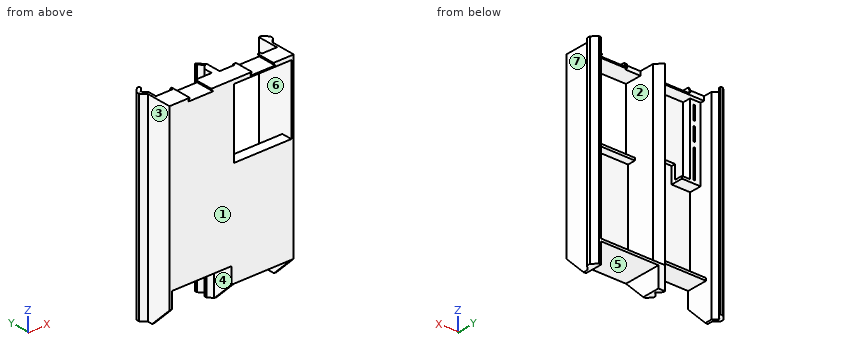
```python
from build123d import *

# Parameters (mm, degrees)
EXTRUDE_1_DEPTH       = 200
SKETCH_2_W            = 148
SKETCH_2_H            = 194
CUT_EXTRUDE_1_DEPTH   = 44
SKETCH_3_W            = 8
SKETCH_3_H            = 194
EXTRUDE_1_2_DEPTH     = 44
CUT_EXTRUDE_2_DEPTH   = 222.580685079
CUT_EXTRUDE_3_DEPTH   = 219.876677606
MOVE_FACE_1_BY        = 2
MOVE_FACE_1_2_BY      = 2
CUT_EXTRUDE_4_DEPTH   = 222.580685079
CUT_EXTRUDE_5_DEPTH   = 16.171573
MOVE_FACE_2_BY        = 45
MOVE_START            = -217
MOVE_FACE_4_DEPTH     = 20
SKETCH_10_W           = 71
SKETCH_10_H           = 47
CUT_EXTRUDE_6_DEPTH   = 25
SKETCH_11_W           = 69
SKETCH_11_H           = 26
CUT_EXTRUDE_7_DEPTH   = 45
CUT_EXTRUDE_8_DEPTH   = 45
CHAMFER_1_SIZE        = 25
CUT_EXTRUDE_9_REACH   = 264.393
SKETCH_13_W           = 71
SKETCH_13_H           = 85
SKETCH_14_W           = 71
SKETCH_14_H           = 3
EXTRUDE_2_DEPTH       = 10
CUT_EXTRUDE_10_DEPTH  = 16.171572875
SKETCH_16_W           = 18.7
SKETCH_16_H           = 5
CUT_EXTRUDE_11_DEPTH  = 4.2
SKETCH_17_W           = 69
SKETCH_17_H           = 90
EXTRUDE_3_DEPTH       = 15
SKETCH_18_W           = 56
SKETCH_18_H           = 87
CUT_EXTRUDE_12_DEPTH  = 10
CUT_EXTRUDE_13_REACH  = 262.298
SKETCH_19_W           = 36
SKETCH_19_H           = 34
SKETCH_21_W           = 2
SKETCH_21_H           = 17
SKETCH_21_H_2         = 35
CUT_EXTRUDE_1_2_DEPTH = 7
MOVE_FACE_5_BY        = 3


# Read off the part's stored shape, not the designer's step: 移动面4
with BuildPart() as part:
    # 草图1 → Extrude 1 (new body)
    with BuildSketch(Plane.XY):
        Polygon((77, 0), (-77, 0), (-77, 31), (-83, 37), (-83, 41), (-77, 47), (77, 47), (83, 41), (83, 37), (77, 31), align=None)
    extrude(amount=-EXTRUDE_1_DEPTH)

    # 草图2 → Cut-Extrude 1 (cut)
    with BuildSketch(Plane(origin=(0, 47, 0), x_dir=(1, 0, 0), z_dir=(0, 1, 0))):
        with Locations((0, 100)):
            Rectangle(SKETCH_2_W, SKETCH_2_H)
    extrude(amount=-CUT_EXTRUDE_1_DEPTH, mode=Mode.SUBTRACT)

    # 草图3 → Extrude 1 2 (add)
    with BuildSketch(Plane(origin=(0, 3, 0), x_dir=(1, 0, 0), z_dir=(0, 1, 0))):
        with Locations((-1, 100)):
            Rectangle(SKETCH_3_W, SKETCH_3_H)
    extrude(amount=EXTRUDE_1_2_DEPTH)

    # 草图6 → 切除-拉伸2 (cut, through all)
    with BuildSketch(Plane.XY):
        Polygon((-74, 47), (-74, 44.343145751), (-79, 39.343145751), (-79, 38.656854249), (-74, 33.656854249), (-74, 26), (-5, 26), (-5, 33.656854249), (0, 38.656854249), (0, 39.343145751), (-5, 44.343145751), (-5, 47), align=None)
    extrude(amount=-CUT_EXTRUDE_2_DEPTH, mode=Mode.SUBTRACT)

    # 草图7 → 切除-拉伸3 (cut, through all)
    with BuildSketch(Plane.XY.offset(-197)):
        Polygon((-4.828427125, 47), (3, 39.171572875), (74, 39.171572875), (74, 47), (3, 47), align=None)
    extrude(amount=CUT_EXTRUDE_3_DEPTH, mode=Mode.SUBTRACT)

    # Move Face 1: a face moved outward by 2.0
    extrude(part.faces().sort_by_distance((-39.5, 14.5, -3))[0], amount=MOVE_FACE_1_BY, dir=(0, 0, -1))

    # Move Face 1 2: a face moved outward by 2.0
    extrude(part.faces().sort_by_distance((38.5, 21.085786438, -3))[0], amount=MOVE_FACE_1_2_BY, dir=(0, 0, -1))

    # 草图8 → 切除-拉伸4 (cut, through all)
    with BuildSketch(Plane.XZ):
        Polygon((-51.883419246, 0), (-53.904145188, -3.5), (-23.095854812, -3.5), (-25.116580754, 0), align=None)
        Polygon((25.116580754, 0), (51.883419246, 0), (53.904145188, -3.5), (23.095854812, -3.5), align=None)
    extrude(amount=-CUT_EXTRUDE_4_DEPTH, mode=Mode.SUBTRACT)

    # 草图9 → 切除-拉伸5 (cut)
    with BuildSketch(Plane(origin=(0, 39.171572875, 0), x_dir=(1, 0, 0), z_dir=(0, 1, 0))):
        Polygon((26.616580754, 0), (24.595854812, 3.5), (55.404145188, 3.5), (53.383419246, 0), (74, 0), (74, 5), (3, 5), (3, 0), align=None)
        Polygon((-55.404145188, 3.5), (-24.595854812, 3.5), (-26.616580754, 0), (-5, 0), (-5, 5), (-74, 5), (-74, 0), (-53.383419246, 0), align=None)
    extrude(amount=-CUT_EXTRUDE_5_DEPTH, mode=Mode.SUBTRACT)

    # Move Face 2: a face moved outward by 45.0
    extrude(part.faces().sort_by_distance((10.164079255, 20.448401084, -200))[0], amount=MOVE_FACE_2_BY, dir=(0, 0, -1))

    # Move Face 4 outline → Move Face 4 (cut)
    with BuildSketch(Plane.XY.offset(MOVE_START)):
        Polygon((74, 3), (74, 47), (-4.828427125, 47), (3, 39.171572875), (3, 3), align=None)
    extrude(amount=MOVE_FACE_4_DEPTH, mode=Mode.SUBTRACT)

    # 草图10 → 切除-拉伸6 (cut)
    with BuildSketch(Plane(origin=(0, 0, -245), x_dir=(-1, 0, 0), z_dir=(0, 0, -1))):
        with Locations((-38.5, 23.5)):
            Rectangle(SKETCH_10_W, SKETCH_10_H)
    extrude(amount=-CUT_EXTRUDE_6_DEPTH, mode=Mode.SUBTRACT)

    # 草图11 → 切除-拉伸7 (cut)
    with BuildSketch(Plane(origin=(0, 0, -245), x_dir=(-1, 0, 0), z_dir=(0, 0, -1))):
        with Locations((39.5, 13)):
            Rectangle(SKETCH_11_W, SKETCH_11_H)
    extrude(amount=-CUT_EXTRUDE_7_DEPTH, mode=Mode.SUBTRACT)

    # 草图12 → 切除-拉伸8 (cut)
    with BuildSketch(Plane(origin=(0, 0, -245), x_dir=(-1, 0, 0), z_dir=(0, 0, -1))):
        Polygon((5, 0), (0, 0), (0, 25.656854249), (5, 30.656854249), align=None)
    extrude(amount=-CUT_EXTRUDE_8_DEPTH, mode=Mode.SUBTRACT)

    # 倒角1
    chamfer_1_edges = [part.edges().sort_by_distance(p)[0] for p in [
        (-75.5, 0, -245),
        (1.5, 0, -245),
        (75.5, 0, -245),
    ]]
    chamfer(chamfer_1_edges, length=CHAMFER_1_SIZE)

    # 草图13 → 切除-拉伸9 (cut, up to next)
    with BuildSketch(Plane(origin=(0, 3, 0), x_dir=(1, 0, 0), z_dir=(0, 1, 0)), mode=Mode.PRIVATE) as cut_extrude_9_sk1:
        with Locations((38.5, 47.5)):
            Rectangle(SKETCH_13_W, SKETCH_13_H)
    cut_extrude_9_tool1 = extrude(cut_extrude_9_sk1.sketch, amount=-CUT_EXTRUDE_9_REACH, mode=Mode.PRIVATE) & part.part
    add(cut_extrude_9_tool1.solids().sort_by_distance((38.5, 3, -47.5))[0], mode=Mode.SUBTRACT)

    # 草图14 → 凸台-拉伸2 (add)
    with BuildSketch(Plane(origin=(0, 3, 0), x_dir=(1, 0, 0), z_dir=(0, 1, 0))):
        with Locations((38.5, 91.5)):
            Rectangle(SKETCH_14_W, SKETCH_14_H)
    extrude(amount=EXTRUDE_2_DEPTH)

    # 草图15 → 切除-拉伸10 (cut)
    with BuildSketch(Plane(origin=(0, 39.171572875, 0), x_dir=(1, 0, 0), z_dir=(0, 1, 0))):
        Polygon((51.883419246, 0), (53.904145188, 3.5), (55.404145188, 3.5), (53.383419246, 0), align=None)
    extrude(amount=-CUT_EXTRUDE_10_DEPTH, mode=Mode.SUBTRACT)

    # 草图16 → 切除-拉伸11 (cut)
    with BuildSketch(Plane(origin=(0, 25, 0), x_dir=(1, 0, 0), z_dir=(0, 1, 0))):
        with Locations((12.35, 2.5)):
            Rectangle(SKETCH_16_W, SKETCH_16_H)
        with Locations((64.65, 2.5)):
            Rectangle(SKETCH_16_W, SKETCH_16_H)
    extrude(amount=-CUT_EXTRUDE_11_DEPTH, mode=Mode.SUBTRACT)

    # 草图17 → 凸台-拉伸3 (add)
    with BuildSketch(Plane(origin=(0, 3, 0), x_dir=(1, 0, 0), z_dir=(0, 1, 0))):
        with Locations((-39.5, 50)):
            Rectangle(SKETCH_17_W, SKETCH_17_H)
    extrude(amount=EXTRUDE_3_DEPTH)

    # 草图18 → 切除-拉伸12 (cut)
    with BuildSketch(Plane(origin=(0, 18, 0), x_dir=(1, 0, 0), z_dir=(0, 1, 0))):
        with Locations((-33, 48.5)):
            Rectangle(SKETCH_18_W, SKETCH_18_H)
    extrude(amount=-CUT_EXTRUDE_12_DEPTH, mode=Mode.SUBTRACT)

    # 切除-拉伸13: up to this face of the body (flat: up to its plane)
    cut_extrude_13_end = Plane(part.part.faces().sort_by_distance((-39.5, 3, -146))[0])
    # 草图19 → 切除-拉伸13 (cut, up to the picked face)
    with BuildSketch(Plane(origin=(0, 18, 0), x_dir=(1, 0, 0), z_dir=(0, 1, 0)), mode=Mode.PRIVATE) as cut_extrude_13_sk1:
        with Locations((-33, 92)):
            Rectangle(SKETCH_19_W, SKETCH_19_H)
    cut_extrude_13_tool1 = split(extrude(cut_extrude_13_sk1.sketch, amount=-CUT_EXTRUDE_13_REACH, mode=Mode.PRIVATE), bisect_by=cut_extrude_13_end, keep=Keep.BOTH, mode=Mode.PRIVATE)
    add(cut_extrude_13_tool1.solids().sort_by(Axis((-33, 18, -92), (0, -1, 0)))[0], mode=Mode.SUBTRACT)

    # 草图21 → Cut-Extrude 1 2 (cut)
    with BuildSketch(Plane(origin=(0, 18, 0), x_dir=(1, 0, 0), z_dir=(0, 1, 0))):
        with Locations((-66, 18.5)):
            Rectangle(SKETCH_21_W, SKETCH_21_H)
        with Locations((-66, 41.5)):
            Rectangle(SKETCH_21_W, SKETCH_21_H)
        with Locations((-66, 73.5)):
            Rectangle(SKETCH_21_W, SKETCH_21_H_2)
    extrude(amount=-CUT_EXTRUDE_1_2_DEPTH, mode=Mode.SUBTRACT)

    # Move Face 5: a face moved outward by 3.0
    extrude(part.faces().sort_by_distance((-66, 11, -73.5))[0], amount=MOVE_FACE_5_BY, dir=(0, 1, 0))


solid = part.part
```
Input: part model. Units: mm. Frame: model coordinates. Face numbers are marked on the shaded views. A direction names the side the tool comes from. Coordinates: 2 decimals unless noted, no trailing zeros. Loops run counter-clockwise (first coordinate to the right, second up) from the corner with the lowest first, then second, coordinate; pieces in that order, holes last. Notation, with made-up numbers: M -10,63 L 6,63 A31 cw 6,89 Z; hole C 73.5,66.25 d11. An arc over 180 degrees is marked long. Use a Markdown table: item, result. Add a question column.
1) Draft query along X for the marked faces 1, 2 and 3. Return one class per face: +X half, -X half, draft (parallel to the pull), parting line (faces both ways), or undercut.
2) Section A-A, the plane z = -148. Return the cut outline in (x, y).
3) Line query: L1, parallel to X at y = 23.5, z = -159; L2, parallel to Z at x = 11.5, y = 8; L3, parallel to Z at x = 54, y = 19.5. Output: solid intervals per line, ascending. Write a range as from..to.
4) Pin query (flat end, axial travel): P1, Ø3.5, axis at x = -9.5, z = -93, coming from the +Y side; P2, Ø3, axis at x = -54, y = 13.5, coming from the +Z side; P3, Ø1, axis at y = 6.5, z = -166.5, coming from the +X side; P4, Ø8, axis at x = -18, y = 32.5, coming from the -Z side. Return the tip coordinate at first contact, or that it passes through.
5) Set-up query: the marked faces 4, 5, 6 and 7. Return all of +Z, -Z, +X, -X, +Y, -Y with unobstructed straight access to the full face (end or side cutting, diameter ignored); none if empty.
Answer below:
| question | item | result |
|---|---|---|
| 1 | face 1 | draft |
| 1 | face 2 | undercut |
| 1 | face 3 | -X half |
| 2 | outline | M -83,37 L -77,31 L -77,0 L 77,0 L 77,31 L 83,37 L 83,41 L 77,47 L 74,47 L 74,3 L 3,3 L 3,39.17 L -4.83,47 L -5,47 L -5,44.34 L 0,39.34 L 0,38.66 L -5,33.66 L -5,3 L -74,3 L -74,33.66 L -79,38.66 L -79,39.34 L -74,44.34 L -74,47 L -77,47 L -83,41 Z |
| 3 | L1 | -77..-74, -5..3, 74..77 |
| 3 | L2 | -220..-217, -93..-90, -5..0 |
| 3 | L3 | -220..-217, -5..0 |
| 4 | P1 | y = 18 |
| 4 | P2 | z = 0 |
| 4 | P3 | x = 77 |
| 4 | P4 | through |
| 5 | face 4 | -Z, -Y |
| 5 | face 5 | -Z, +Y, -Y |
| 5 | face 6 | +Y |
| 5 | face 7 | +Z, -Z, +X, -Y |
